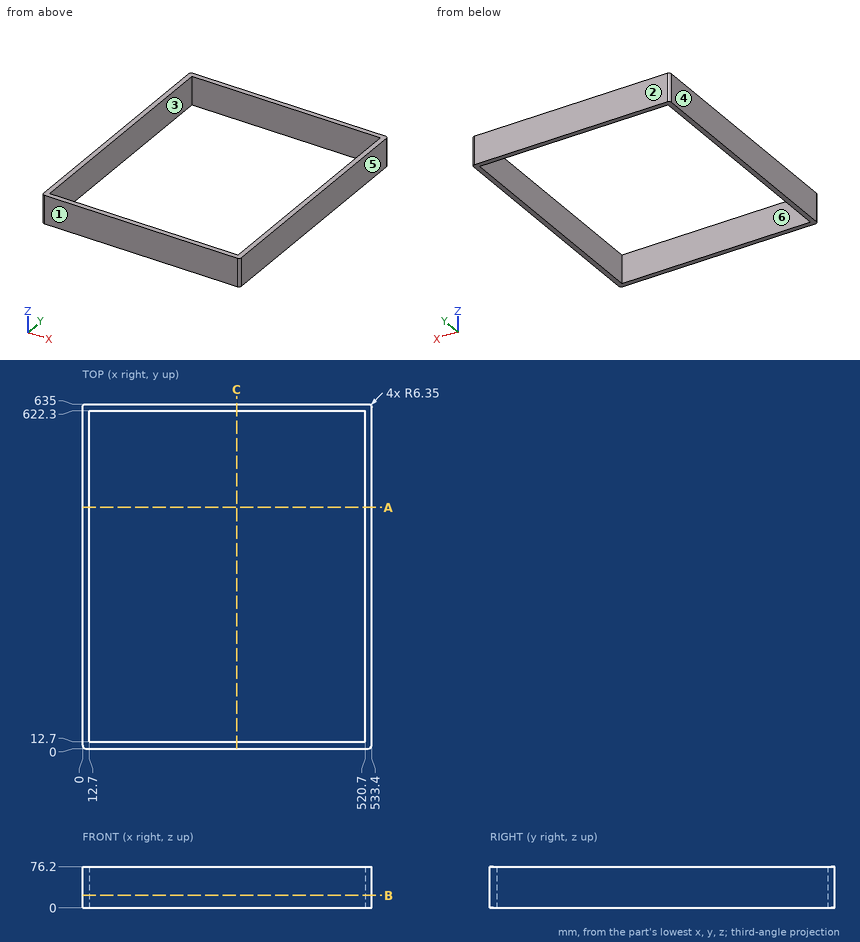
Geometry: see drawing. Coordinates: mm, zero at the bounding-box minimum. A direction names the side the tool comes from. Coordinates: 2 decimals unless noted, no trailing zeros. Loops run counter-clockwise (first coordinate to the right, second up) from the corner with the lowest first, then second, coordinate; pieces in that order, holes last. Notation, with made-up numbers: (47, 52.5) - (63, 52.5) arc R12 ccw to (63, 62.5) - close; hole circle Ø1 at (57, 65). An arc over 180 degrees is marked (long way). Answer as CSV lines item,"result".
1. Ray query, line 1 (Y direction, x = 281, z = 51); line 2 (X direction, y = 90, z = 16.5). Return the intervals inside material, ascending.
Established:
line 1,"y = 0 to 12.7, 622.3 to 635"
line 2,"x = 0 to 12.7, 520.7 to 533.4"
2. Section A-A (y = 444.5). Return loops of the section in (x, z).
Established:
outline,"(0, 0) - (12.7, 0) - (12.7, 76.2) - (0, 76.2) - close; (520.7, 0) - (533.4, 0) - (533.4, 76.2) - (520.7, 76.2) - close"
3. Section C-C (x = 284). Return loops of the section in (y, z).
Established:
outline,"(0, 0) - (12.7, 0) - (12.7, 76.2) - (0, 76.2) - close; (622.3, 0) - (635, 0) - (635, 76.2) - (622.3, 76.2) - close"
4. Reachability of the marked faces 5 and 6 from +Z, -Z, +X, -X, +Y, -Y: full face, straight path, thin tool, end or side. Return the list, or none.
Established:
face 5,"+Z, -Z, +X, +Y, -Y"
face 6,"+Z, -Z"
5. Mould query, pull axis Y, two halves, no side actions, for the marked faces 1, 2, 3 and 4. Classes: released by +Y, released by -Y, zero draft, split by the parting line, or undercut.
Established:
face 1,"released by -Y"
face 2,"released by +Y"
face 3,"undercut"
face 4,"zero draft"
6. Section B-B (z = 23). Return loops of the section in (x, y).
Established:
outline,"(0, 6.35) arc R6.35 ccw to (6.35, 0) - (527.05, 0) arc R6.35 ccw to (533.4, 6.35) - (533.4, 628.65) arc R6.35 ccw to (527.05, 635) - (6.35, 635) arc R6.35 ccw to (0, 628.65) - close; hole (12.7, 12.7) - (520.7, 12.7) - (520.7, 622.3) - (12.7, 622.3) - close"
